Geometry check sheet. Reference: drawing and pictorial views, mm from the part's lowest x, y, z. Give positions to 0.01 mm unless a question says otherwise; leave off trailing zeros. Loops run counter-clockwise (first coordinate to the right, second up) from the corner with the lowest first, then second, coordinate; pieces in that order, holes last. Notation, with made-up numbers: (11, 17) - (59, 17) arc R8 ccw to (59, 21) - close; hole circle Ø11 at (-40, 52.25). An arc over 180 degrees is marked (long way). Answer in a Markdown table with one row per item. Add a question column.
(1) Sectioned sample at C-C on z = 756.5. Enter the section's corners in (x, y).
(2) Sectioned sample at A-A on x = 155.5. Enter the section's corners in (y, z).
(3) Thickness scan on L1, parallel to Z at x = 130, y = 246; L2, parallel to X at y = 147, z = 1376.5; L3, parallel to Y at x = 148.5, z = 714.5. Record the ranges inside material, lowest first.
(4) Sectioned sample at D-D on x = 228. Enter the section's corners in (y, z), then the cut area to 3 significant figures.
(5) Sectioned sample at B-B on y = 108. Enter the section's corners in (x, z).
(6) Go/stop test with flat-tipped pins: P1, Ø15.5, axis at y = 259, z = 174.5, coming from the +X side; P2, Ø16.5, axis at x = 146.5, y = 267, coming from the -Z side; P3, Ø6, axis at x = 247.5, y = 78.5, coming from the -Z side; P4, Ø2, axis at x = 237, z = 556.5, coming from the +Y side. Record where each tip stops, or that it passes through.
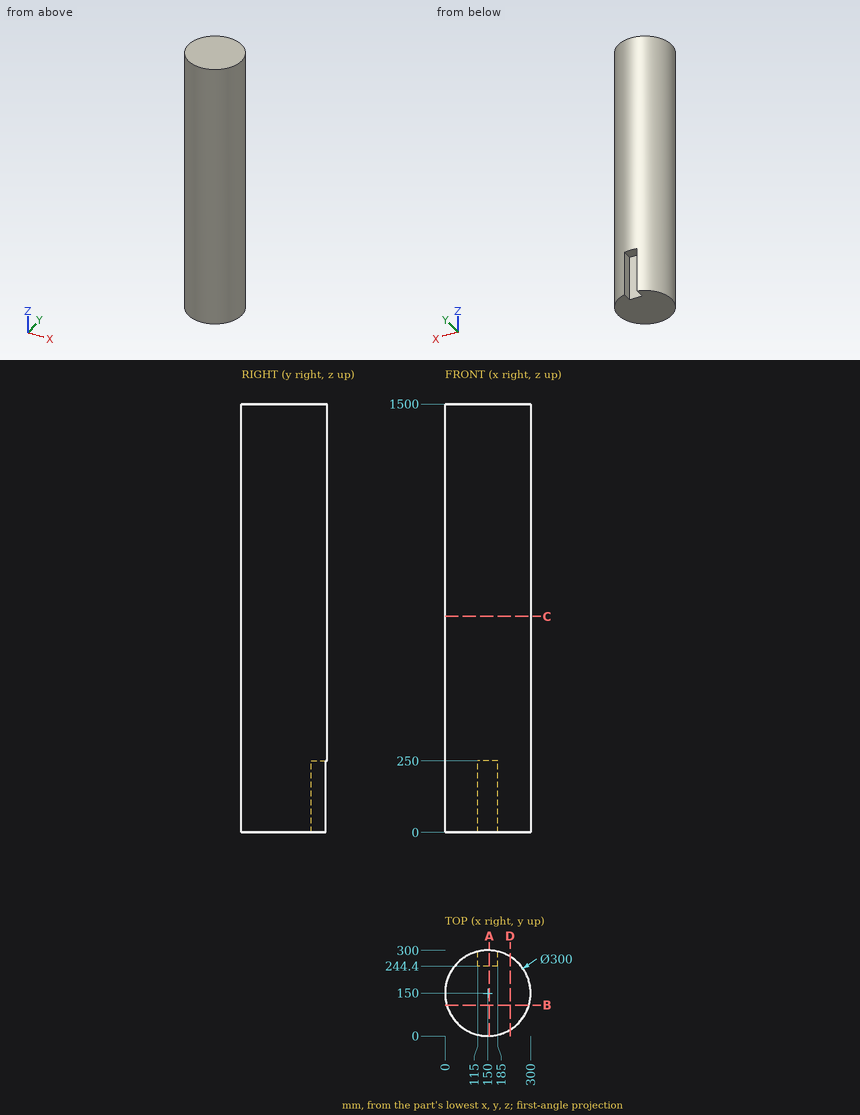
Reply:
| question | item | result |
|---|---|---|
| 1 | outline | circle Ø300 at (150, 150) |
| 2 | outline | (0.1, 0) - (244.4, 0) - (244.4, 250) - (299.9, 250) - (299.9, 1500) - (0.1, 1500) - close |
| 3 | L1 | 250 to 1500 |
| 3 | L2 | 0.03 to 299.97 |
| 3 | L3 | 0.01 to 299.99 |
| 4 | outline | (21.88, 0) - (278.12, 0) - (278.12, 1500) - (21.88, 1500) - close |
| 4 | area | 384,000 mm^2 |
| 5 | outline | (6, 0) - (294, 0) - (294, 1500) - (6, 1500) - close |
| 6 | P1 | x = 260.67 |
| 6 | P2 | z = 250 |
| 6 | P3 | z = 0 |
| 6 | P4 | y = 272.9 |
